Geometry check sheet. Reference: drawing and pictorial views, mm from the part's lowest x, y, z. A direction names the side the tool comes from. Coordinates: 2 decimals unless noted, no trailing zeros. Write each loop counter-clockwise with the first axis right and the second up, starting at its lowest first coordinate (ties: lowest second). Pieces come first, ordered by that corner, then holes. Notation, with made-up numbers: (23, 73) -> (70, 73) arc R24 ccw to (70, 89) -> close; hole circle Ø8 at (22, -21.75). An arc over 180 degrees is marked (long way). Answer in a Markdown table with one row per item.
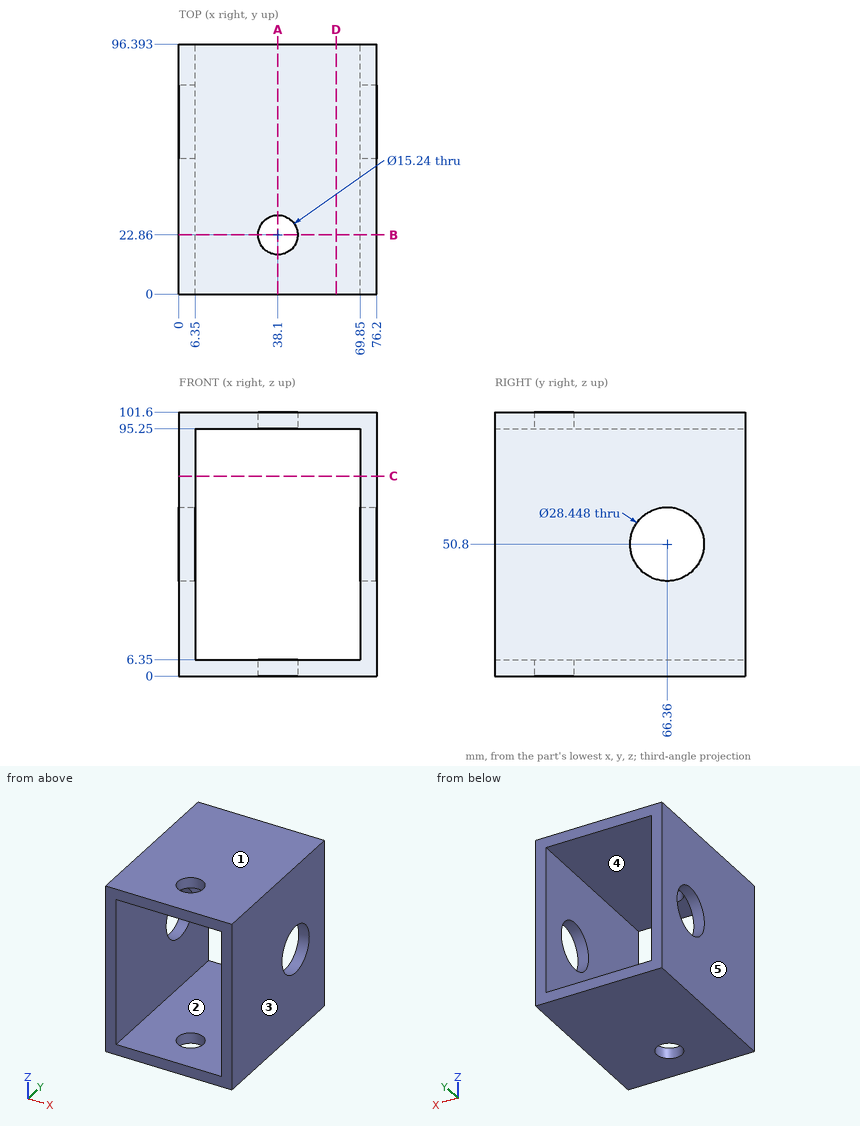
1. Section check A-A, the plane x = 38.1. Record the boundary of the cut face in (y, z), plus the area to 3 significant figures.
Geometry says:
| item | result |
|---|---|
| outline | (0, 0) -> (15.24, 0) -> (15.24, 6.35) -> (0, 6.35) -> close; (0, 95.25) -> (15.24, 95.25) -> (15.24, 101.6) -> (0, 101.6) -> close; (30.48, 0) -> (96.39, 0) -> (96.39, 6.35) -> (30.48, 6.35) -> close; (30.48, 95.25) -> (96.39, 95.25) -> (96.39, 101.6) -> (30.48, 101.6) -> close |
| area | 1,030 mm^2 |
2. Section check D-D, the plane x = 60.5. Record the boundary of the cut face in (y, z).
Geometry says:
| item | result |
|---|---|
| outline | (0, 0) -> (96.39, 0) -> (96.39, 6.35) -> (0, 6.35) -> close; (0, 95.25) -> (96.39, 95.25) -> (96.39, 101.6) -> (0, 101.6) -> close |
3. Section check B-B, the plane y = 22.86. Record the boundary of the cut face in (x, z).
Geometry says:
| item | result |
|---|---|
| outline | (0, 0) -> (30.48, 0) -> (30.48, 6.35) -> (6.35, 6.35) -> (6.35, 95.25) -> (30.48, 95.25) -> (30.48, 101.6) -> (0, 101.6) -> close; (45.72, 0) -> (76.2, 0) -> (76.2, 101.6) -> (45.72, 101.6) -> (45.72, 95.25) -> (69.85, 95.25) -> (69.85, 6.35) -> (45.72, 6.35) -> close |
4. Thickness scan on line 1 (Z direction, x = 17, y = 7.5); line 2 (Y direction, x = 74, z = 50); line 3 (X direction, y = 76.5, z = 19). Record the ranges inside material, lowest first. Write a range as from..to.
Geometry says:
| item | result |
|---|---|
| line 1 | 0..6.35, 95.25..101.6 |
| line 2 | 0..52.16, 80.56..96.39 |
| line 3 | 0..6.35, 69.85..76.2 |
5. Tool access check on the marked faces 4 and 5. Record the directions out of +Z, -Z, +X, -X, +Y, -Y that give a thin tool (end or side, any length) a straight path to the whole face; none if there is none.
Geometry says:
| item | result |
|---|---|
| face 4 | +Y, -Y |
| face 5 | +Z, -Z, -X, +Y, -Y |
6. Mould release check, pull along Z, two halves, no side actions. Record for the marked faces 1, 2 and 3: released by +Z, released by -Z, zero draft, split by the parting line, or undercut.
Geometry says:
| item | result |
|---|---|
| face 1 | released by +Z |
| face 2 | undercut |
| face 3 | zero draft |
7. Section check C-C, the plane z = 77. Record the boundary of the cut face in (x, y).
Geometry says:
| item | result |
|---|---|
| outline | (0, 0) -> (6.35, 0) -> (6.35, 96.39) -> (0, 96.39) -> close; (69.85, 0) -> (76.2, 0) -> (76.2, 96.39) -> (69.85, 96.39) -> close |
